Here's how the part is built. I have some questions about the finished solid (model axes, mm). A direction names the side the tool comes from. Coordinates: 2 decimals unless noted, no trailing zeros. Write each loop counter-clockwise with the first axis right and the second up, starting at its lowest first coordinate (ties: lowest second). Pieces come first, ordered by that corner, then holes.
(1) Imagine slicing it at A-A, the plane x = 12. List the corners of the cut face in (y, z) for me.
(2) Which directions (+Z, -Z, +X, -X, +Y, -Y) give clear straight access to the entire face, cutting with the end or side of a thin tool? Please do faces 1 (the flat face through (10, -15.775, 1)), 2 (the flat face through (3.094, 3, 1)), 3 (the flat face through (8, 1.154, 1)), 4 (the flat face through (12.428, 3, 1)).
(3) Imagine slicing it at C-C, the plane x = 5. List the corners of the cut face in (y, z) for me.
(4) For pin 1 Ø0.8 at (x, z) = (2.5, 1) entering from +Y; pin 2 Ø1 at (y, z) = (2.5, 1.5) entering from -X; pin 3 Ø3 at (x, y) = (11.5, -12) entering from +Z; pin 4 Ø0.6 at (y, z) = (-14.5, 0.5) entering from +X, each with a flat end and sliding along its axis, tell me the tip position at first contact or that it passes through.
(5) Please list where these lines run through material, in increasing order: probe 1 along Y at (x, z) = (6.75, 1.8); probe 2 along Y at (x, z) = (12.5, 0.35); probe 3 along X at (y, z) = (4.25, 1.6).
(6) Thinking about a two-plate mould opening in Y: for faces 5 (the flat face through (10, -10.895, 1)), 6 (the flat face through (5, -6, 0)), 7 (the flat face through (8, -19.089, 1)), 8 (the flat face through (8, 6.866, 1)), which applies, released by +Y, released by -Y, zero draft, split by the parting line, or undercut?
(7) Imagine slicing it at D-D, the plane x = 9.75. List the corners of the cut face in (y, z) for me.
(8) Imagine slicing it at B-B, the plane y = 4. List the corners of the cut face in (x, z) for me.
```python
from build123d import *

# Parameters (mm, degrees)
F0_W     = 4.4058337156
F0_H     = 0.9129986805
F0_W_2   = 4.9275004491
F1_DEPTH = 2


with BuildPart() as f1:
    # F0 (on Top) → F1 (new body)
    with BuildSketch(Plane.XY):
        with Locations((5.2970831422, -0.618056921)):
            Rectangle(F0_W, F0_H)
        Polygon((7.5, -1.0745562613), (3.0941662844, -1.0745562613), (3.0941662844, -0.1615575808), (2.381938691, -0.1615575808), (2.381938691, -19.0886495443), (13.2808616404, -19.0886495443), (13.2808616404, -15.7746478873), (6.396023198, -15.7746478873), (6.396023198, -10.8947804474), (12.8044739022, -10.8947804474), (12.8044739022, -7.6056338028), (6.396023198, -7.6056338028), (6.396023198, -3.4507042254), (13.2808616404, -3.4507042254), (13.2808616404, -0.1615575808), (12.4275004491, -0.1615575808), (12.4275004491, -1.0745562613), align=None)
        with Locations((9.9637502246, -0.618056921)):
            Rectangle(F0_W_2, F0_H)
        Polygon((3.0941662844, 6.8657421507), (3.0941662844, -0.1615575808), (7.5, -0.1615575808), (7.5, 1.1542992434), (4.6620512009, 1.1542992434), (4.6620512009, 4.636886646), (7.5, 4.636886646), (7.5, 6.8657421507), align=None)
        Polygon((7.5, 1.1542992434), (7.5, -0.1615575808), (12.4275004491, -0.1615575808), (12.4275004491, 6.8657421507), (7.5, 6.8657421507), (7.5, 4.636886646), (10.3379487991, 4.636886646), (10.3379487991, 1.1542992434), align=None)
    extrude(amount=F1_DEPTH)


solid = f1.part
```
Recorded:
1. outline: (-19.09, 0) - (-15.77, 0) - (-15.77, 2) - (-19.09, 2) - close; (-10.89, 0) - (-7.61, 0) - (-7.61, 2) - (-10.89, 2) - close; (-3.45, 0) - (6.87, 0) - (6.87, 2) - (-3.45, 2) - close
2. face 1: +Z, -Z, +X
2. face 2: +Z, -Z, -X, +Y
2. face 3: +Z, -Z
2. face 4: +Z, -Z, +X, +Y
3. outline: (-19.09, 0) - (1.15, 0) - (1.15, 2) - (-19.09, 2) - close; (4.64, 0) - (6.87, 0) - (6.87, 2) - (4.64, 2) - close
4. pin 1: stops at y = -0.16
4. pin 2: stops at x = 3.09
4. pin 3: stops at z = 2
4. pin 4: stops at x = 6.4
5. probe 1: y = -19.09 to -15.77, -10.89 to -7.61, -3.45 to 1.15, 4.64 to 6.87
5. probe 2: y = -19.09 to -15.77, -10.89 to -7.61, -3.45 to -0.16
5. probe 3: x = 3.09 to 4.66, 10.34 to 12.43
6. face 5: undercut
6. face 6: zero draft
6. face 7: released by -Y
6. face 8: released by +Y
7. outline: (-19.09, 0) - (-15.77, 0) - (-15.77, 2) - (-19.09, 2) - close; (-10.89, 0) - (-7.61, 0) - (-7.61, 2) - (-10.89, 2) - close; (-3.45, 0) - (1.15, 0) - (1.15, 2) - (-3.45, 2) - close; (4.64, 0) - (6.87, 0) - (6.87, 2) - (4.64, 2) - close
8. outline: (3.09, 0) - (4.66, 0) - (4.66, 2) - (3.09, 2) - close; (10.34, 0) - (12.43, 0) - (12.43, 2) - (10.34, 2) - close
